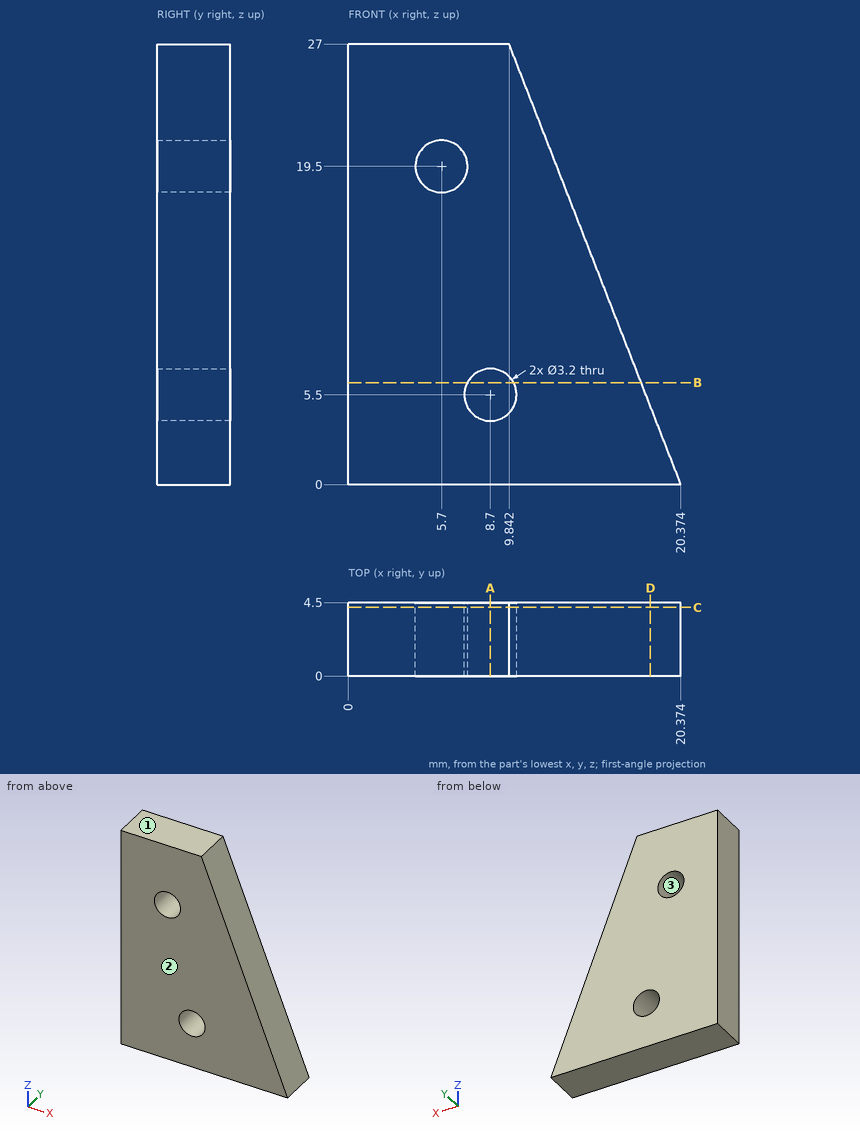
The figure shows three views and two pictorial views of one solid part (mm, origin at its lowest corner). Answer the questions. Coordinates: 2 decimals unless noted, no trailing zeros. Loops run counter-clockwise (first coordinate to the right, second up) from the corner with the lowest first, then second, coordinate; pieces in that order, holes last. Notation, with made-up numbers: (66.5, 76) -> (105.5, 76) arc R7 ccw to (105.5, 85) -> close; hole circle Ø7 at (16.25, -33). An arc over 180 degrees is marked (long way). Return JSON: item names as keys, results as strings. Group by question number.
(1) A cutting plane is placed at B-B on z = 6.25. Write down the section's boundary in (x, y).
(2) A cutting plane is placed at C-C on y = 4.2. Write down the section's boundary in (x, z), and give its area (3 significant figures).
(3) Determine the mould class of the marked faces 1, 2 and 3 for opening direction Z: released by +Z, released by -Z, zero draft, split by the parting line, or undercut.
(4) Find the intervals of material crossed by probe 1 along Z at (x, y) = (8.7, 2.2); probe 2 along X at (y, z) = (3.45, 5.5); probe 3 along Z at (x, y) = (5.7, 2.8), in increasing order. Write a range as from..to.
(5) A cutting plane is placed at A-A on x = 8.7. Write down the section's boundary in (y, z), and give its area (3 significant figures).
(6) A cutting plane is placed at D-D on x = 18.5. Write down the section's boundary in (y, z), and give its area (3 significant figures).
(7) Given pin 1 Ø1 at (y, z) = (3.5, 16.5) entering from +X, flat-ended and moving along its own axis, determine where the tip first touches the part or whether it passes through.
The answers:
{
 "1": {"outline": "(0, 0) -> (7.29, 0) -> (7.29, 4.5) -> (0, 4.5) -> close; (10.11, 0) -> (17.94, 0) -> (17.94, 4.5) -> (10.11, 4.5) -> close"},
 "2": {"outline": "(0, 0) -> (20.37, 0) -> (9.84, 27) -> (0, 27) -> close; hole circle Ø3.2 at (5.7, 19.5); hole circle Ø3.2 at (8.7, 5.5)", "area": "392 mm^2"},
 "3": {"face 1": "released by +Z", "face 2": "zero draft", "face 3": "undercut"},
 "4": {"probe 1": "z = 0..3.9, 7.1..27", "probe 2": "x = 0..7.1, 10.3..18.23", "probe 3": "z = 0..17.9, 21.1..27"},
 "5": {"outline": "(0, 0) -> (4.5, 0) -> (4.5, 3.9) -> (0, 3.9) -> close; (0, 7.1) -> (4.5, 7.1) -> (4.5, 27) -> (0, 27) -> close", "area": "107 mm^2"},
 "6": {"outline": "(0, 0) -> (4.5, 0) -> (4.5, 4.8) -> (0, 4.8) -> close", "area": "21.6 mm^2"},
 "7": {"pin 1": "stops at x = 14.13"}
}
